Source: CAD feature listing. Evaluate the final solid. Frame: model axes, mm. A direction names the side the tool comes from. Give positions to 0.01 mm unless a question says otherwise; leave off trailing zeros. Order: outer loops, then holes, each group sorted by start corner. A loop starts at its lowest first (then second) coordinate and runs counter-clockwise, first axis right, second up. Notation, with made-up numbers: M -23,31.25 L 18,31.25 A25 ccw 18,60.25 Z; hole C 65,-17 d10. An arc over 180 degrees is marked long. Answer in a Markdown table with one row per item. Add a question column.
(1) Section query C-C, the plane x = 0. Return loops of the section in (y, z).
(2) Section query D-D, the plane x = -10.5. Return loops of the section in (y, z), plus the area to 3 significant figures.
(3) Set-up query: faces 4 (the face through (-20, -2, 1)), 5 (the face through (-43.5, -0.1, 1.5)), 6 (the face through (-36.2, 2.29, 1.48)). Return all of +Z, -Z, +X, -X, +Y, -Y with unobstructed straight access to the full face (end or side cutting, diameter ignored); none if empty.
(4) Section query A-A, the plane y = 0. Return loops of the section in (x, z).
(5) Section query B-B, the plane z = 2.4. Return loops of the section in (x, y), plus the area to 3 significant figures.
(6) Mould query, pull axis Z, two halves, no side actions, for faces 1 (the face through (-20, 0, 3)), 2 (the face through (-20, 0, 0)), 3 (the face through (-20, 2, 1)). Classes: pulls with the +Z half, pulls with the -Z half, needs draft (parallel to the pull), parting line crosses it, or undercut.
(7) Pin query (flat end, axial travel): P1, Ø1, axis at x = -24, z = 2, coming from the +Y side; P2, Ø3.5, axis at x = 0, y = 0, coming from the +Z side. Return the tip coordinate at first contact, or that it passes through.
(8) Material intervals for line 1 along Y through (x, z) = (-40, 1.65); line 2 along X through (y, z) = (0.75, 0.3); line 3 along X through (y, z) = (1, 1.2), sorted ascending.
from build123d import *

# Parameters (mm, degrees)
SKETCH1_R           = 1.5
BOSS_EXTRUDE1_DEPTH = 3


with BuildPart() as part:
    # Sketch1 → Boss-Extrude1 (new body)
    with BuildSketch(Plane.XY):
        with BuildLine():
            Line((-33.815341562, 2), (-6.184658438, 2))
            ThreePointArc((-6.184658438, 2), (-3.827635834, 2.281746842), (-1.603429966, 3.111111111))
            ThreePointArc((-1.603429966, 3.111111111), (3.5, 0), (-1.603429966, -3.111111111))
            ThreePointArc((-1.603429966, -3.111111111), (-3.827635834, -2.281746842), (-6.184658438, -2))
            Line((-6.184658438, -2), (-33.815341562, -2))
            ThreePointArc((-33.815341562, -2), (-36.172364166, -2.281746842), (-38.396570034, -3.111111111))
            ThreePointArc((-38.396570034, -3.111111111), (-43.5, 0), (-38.396570034, 3.111111111))
            ThreePointArc((-38.396570034, 3.111111111), (-36.172364166, 2.281746842), (-33.815341562, 2))
        make_face()
        Circle(SKETCH1_R, mode=Mode.SUBTRACT)
        with Locations(Location((-40, 0, 0), (0, 0, 180))):
            Circle(SKETCH1_R, mode=Mode.SUBTRACT)
    extrude(amount=BOSS_EXTRUDE1_DEPTH)


solid = part.part
Values follow:
| question | item | result |
|---|---|---|
| 1 | outline | M -3.5,0 L -1.5,0 L -1.5,3 L -3.5,3 Z; M 1.5,0 L 3.5,0 L 3.5,3 L 1.5,3 Z |
| 2 | outline | M -2,0 L 2,0 L 2,3 L -2,3 Z |
| 2 | area | 12.0 mm² |
| 3 | face 4 | +Z, -Z, -Y |
| 3 | face 5 | +Z, -Z |
| 3 | face 6 | +Z, -Z, +Y |
| 4 | outline | M -43.5,0 L -41.5,0 L -41.5,3 L -43.5,3 Z; M -38.5,0 L -1.5,0 L -1.5,3 L -38.5,3 Z; M 1.5,0 L 3.5,0 L 3.5,3 L 1.5,3 Z |
| 5 | outline | M -38.4,-3.11 A10 cw -33.82,-2 L -6.18,-2 A10 cw -1.6,-3.11 A3.5 ccw long -1.6,3.11 A10 cw -6.18,2 L -33.82,2 A10 cw -38.4,3.11 A3.5 ccw long Z; hole C -40,0 d3; hole C 0,0 d3 |
| 5 | area | 200 mm² |
| 6 | face 1 | pulls with the +Z half |
| 6 | face 2 | pulls with the -Z half |
| 6 | face 3 | needs draft |
| 7 | P1 | stops at y = 2 |
| 7 | P2 | stops at z = 3 |
| 8 | line 1 | y = -3.5 to -1.5, 1.5 to 3.5 |
| 8 | line 2 | x = -43.42 to -41.3, -38.7 to -1.3, 1.3 to 3.42 |
| 8 | line 3 | x = -43.35 to -41.12, -38.88 to -1.12, 1.12 to 3.35 |
